Check sheet for the modelled part. Datum: model origin and axes. Units: mm. A direction names the side the tool comes from. Round coordinates to 2 decimals unless told otherwise and drop trailing zeros. Order: outer loops, then holes, each group sorted by start corner. A loop starts at its lowest first (then second) coordinate and runs counter-clockwise, first axis right, second up.
Q1. Depth check by flat-ended pin: P1, Ø1, axis at x = 2.5, y = 14.5, coming from the -Z side; P2, Ø4, axis at x = 2.5, z = -0.5, coming from the -Y side; P3, Ø3, axis at x = 2.5, y = 10, coming from the +Z side. Enter the tip coordinate at first touch or a pass-through.
Q2. Scan lines: probe 1 along Y at (x, z) = (4, 0); probe 2 along X at (y, z) = (-8, 17.5); probe 3 along Y at (x, z) = (1, -11). Record each from-to range of solid material in increasing order.
Q3. Mould release check, pull along Y, two halves, no side actions. Record for faces 3 (the flat face through (6, -15, 5)), 4 (the cylindrical face through (3.566, -21.086, 4.682)), 5 (the flat face through (0, -15, -5)): +Y half, -Y half, draft (parallel to the pull), parting line (faces both ways), or undercut.
Q4. Cross-section at C-C on x = 4.5. Record the cut outline in (y, z), then the cut area to 3 significant figures.
Q5. Cross-section at A-A on y = 0. Record the cut outline in (x, z), then the cut area to 3 significant figures.
Q6. Set-up check for faces 1 (the cylindrical face through (0.59, -10.54, 11.5)), 2 (the flat face through (1.2, -15, -5)): record each of +Z, -Z, +X, -X, +Y, -Y from which the full face is reachable in a straight line by a thin tool's end or side.
from build123d import *

# Parameters (mm, degrees)
ESQUISSE1_R        = 21.6
ESQUISSE1_R_2      = 20.4
BOSS_EXTRU_3_DEPTH = 7.2
BOSS_EXTRU_4_START = -1.2
ESQUISSE4_R        = 20.4
ESQUISSE4_R_2      = 15.6
BOSS_EXTRU_4_DEPTH = 1.2
ESQUISSE5_R        = 20.4
ESQUISSE5_R_2      = 15.6
BOSS_EXTRU_5_DEPTH = 1.2
CONG_3_R           = 1.2


with BuildPart() as part:
    # Esquisse1 → Boss.-Extru.3 (new body)
    with BuildSketch(Plane(origin=(0, 0, 0), x_dir=(0, 0, -1), z_dir=(1, 0, 0))):
        Circle(ESQUISSE1_R)
        Circle(ESQUISSE1_R_2, mode=Mode.SUBTRACT)
    extrude(amount=BOSS_EXTRU_3_DEPTH)

    # Esquisse4 → Boss.-Extru.4 (add)
    with BuildSketch(Plane(origin=(7.2, 0, 0), x_dir=(0, 0, -1), z_dir=(1, 0, 0)).offset(BOSS_EXTRU_4_START)):
        Circle(ESQUISSE4_R)
        Circle(ESQUISSE4_R_2, mode=Mode.SUBTRACT)
    extrude(amount=BOSS_EXTRU_4_DEPTH)

    # Esquisse5 → Boss.-Extru.5 (add)
    with BuildSketch(Plane.ZY):
        Circle(ESQUISSE5_R)
        with Locations(Location((0, 0, 0), (0, 0, 180))):
            Circle(ESQUISSE5_R_2, mode=Mode.SUBTRACT)
    extrude(amount=-BOSS_EXTRU_5_DEPTH)

    # Congé3
    cong_3_edges = [part.edges().sort_by_distance(p)[0] for p in [
        (0, 0, 21.6),
        (7.2, 0, 21.6),
    ]]
    fillet(cong_3_edges, radius=CONG_3_R)


solid = part.part
Results found:
1. P1: stops at z = -16.45
1. P2: stops at y = -21.6
1. P3: stops at z = 19.86
2. probe 1: y = -21.6 to -20.4, 20.4 to 21.6
2. probe 2: x = 0 to 1.2, 6 to 7.2
2. probe 3: y = -18.57 to -11.06, 11.06 to 18.57
3. face 3: undercut
3. face 4: parting line
3. face 5: draft
4. outline: circle Ø43.2 at (0, 0); hole circle Ø40.8 at (0, 0)
4. area: 158 mm2
5. outline: (0, -20.4) arc R1.2 ccw to (1.2, -21.6) - (6, -21.6) arc R1.2 ccw to (7.2, -20.4) - (7.2, -15.6) - (6, -15.6) - (6, -20.4) - (1.2, -20.4) - (1.2, -15.6) - (0, -15.6) - close; (0, 15.6) - (1.2, 15.6) - (1.2, 20.4) - (6, 20.4) - (6, 15.6) - (7.2, 15.6) - (7.2, 20.4) arc R1.2 ccw to (6, 21.6) - (1.2, 21.6) arc R1.2 ccw to (0, 20.4) - close
5. area: 39.1 mm2
6. face 1: +X, -X
6. face 2: none
